Print and shaded views of the part. All mm, measured from the part's lowest x, y and z. Coordinates: 2 decimals unless noted, no trailing zeros. Loops run counter-clockwise (first coordinate to the right, second up) from the corner with the lowest first, then second, coordinate; pieces in that order, holes last. Notation, with made-up numbers: (-3.5, 21.5) -> (50.5, 21.5) arc R8 ccw to (50.5, 26.5) -> close; hole circle Ø4 at (-24.5, -29). An arc over 180 degrees is marked (long way). One line per item, written item: value. Start each with the question number.
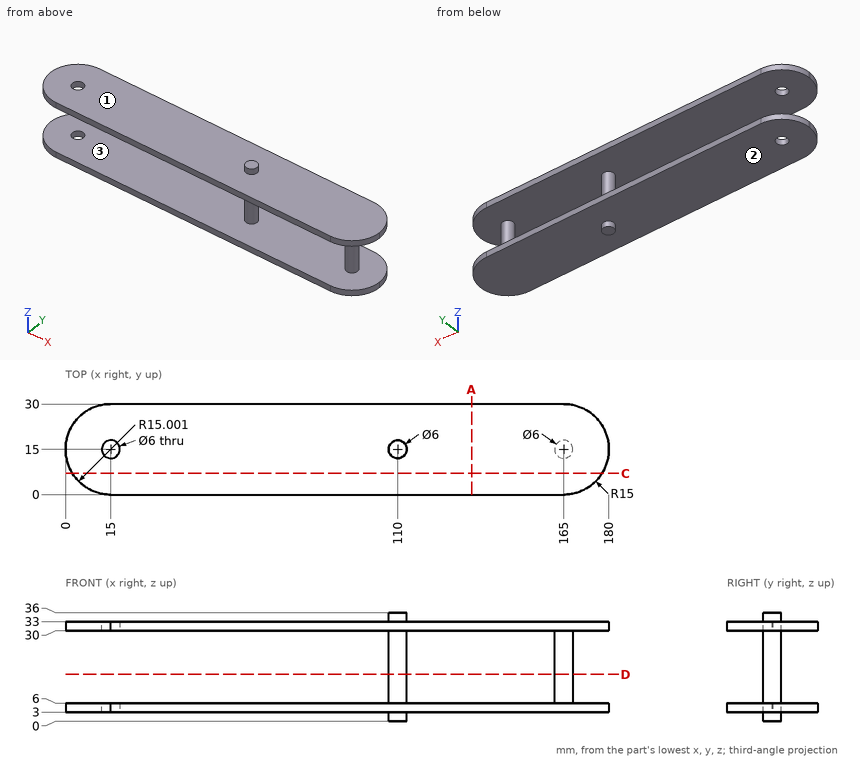
1) Pull direction Z, two halves, no side cores. Call the marked faces 1, 2 and 3: +Z half, -Z half, draft (parallel to the pull), parting line (faces both ways), or undercut.
2) Slice it at D-D (z = 15.5). Give the cut face in (x, y).
3) Probe line 1 (Z direction, x = 83.5, y = 25); line 2 (Y direction, x = 15, z = 31); line 3 (X direction, y = 14, z = 13). List the from-to ranges inside material, lowest first. Write a range as from..to.
4) Slice it at A-A (x = 134.5). Give the cut face in (y, z), then the cut area to 3 significant figures.
5) Slice it at C-C (y = 7). Give the cut face in (x, z).
6) Pin check, flat tips, straight feed: pin 1 Ø7 at (x, y) = (15, 15) entering from -Z; pin 2 Ø1 at (y, z) = (12, 13) entering from +X; pin 3 Ø12 at (y, z) = (16, 23) entering from +X; pin 4 Ø5.5 at (x, y) = (15, 15) entering from +Z. Stop position of each tip, or through.
Check sheet entries:
1. face 1: +Z half
1. face 2: -Z half
1. face 3: undercut
2. outline: circle Ø6 at (110, 15); circle Ø6 at (165, 15)
3. line 1: z = 3..6, 30..33
3. line 2: y = 0..12, 18..30
3. line 3: x = 107.17..112.83, 162.17..167.83
4. outline: (0, 3) -> (30, 3) -> (30, 6) -> (0, 6) -> close; (0, 30) -> (30, 30) -> (30, 33) -> (0, 33) -> close
4. area: 180 mm^2
5. outline: (2.31, 3) -> (177.69, 3) -> (177.69, 6) -> (2.31, 6) -> close; (2.31, 30) -> (177.69, 30) -> (177.69, 33) -> (2.31, 33) -> close
6. pin 1: stops at z = 3
6. pin 2: stops at x = 166.66
6. pin 3: stops at x = 168
6. pin 4: passes through
